```python
from build123d import *

# Parameters (mm, degrees)
SKETCH2_W = 1.05
SKETCH2_H = 10.761
GAP_DEPTH = 3.1


with BuildPart() as part:
    # Sketch1 → Base-Revolve (revolve)
    with BuildSketch(Plane.XY):
        with BuildLine():
            Line((0, 7.1), (0, 10.55))
            Line((0, 10.55), (-2.1, 10.55))
            Line((-2.1, 10.55), (-2.1, 7.1))
            ThreePointArc((-2.1, 7.1), (-1.807106781, 6.392893219), (-1.1, 6.1))
            Line((-1.1, 6.1), (-1, 6.1))
            ThreePointArc((-1, 6.1), (-0.292893219, 6.392893219), (0, 7.1))
        make_face()
    revolve(axis=Axis((-34.925, 0, 0), (1, 0, 0)))

    # Sketch2 → Gap (cut, through all)
    with BuildSketch(Plane(origin=(0, 0, 0), x_dir=(0, -1, 0), z_dir=(-1, 0, 0))):
        with Locations((0, 5.3805)):
            Rectangle(SKETCH2_W, SKETCH2_H)
    extrude(amount=GAP_DEPTH, mode=Mode.SUBTRACT)


solid = part.part
```
Source: CAD feature listing. Evaluate the final solid. Frame: model axes, mm. Coordinates: 2 decimals unless noted, no trailing zeros. Order: outer loops, then holes, each group sorted by start corner. A loop starts at its lowest first (then second) coordinate and runs counter-clockwise, first axis right, second up. Notation, with made-up numbers: M 18.5,36 L 77.5,36 A29 cw 77.5,62 Z; hole C 84.5,53.25 d3. An arc over 180 degrees is marked long. Write each question's results on one line, items separated by ' | '. Start each with the question number.
1) Section query D-D (z = -8). Return the cut outline in (x, y).
2) Draft query along Y for faces 1 (the face through (-1, 0.525, 8)), 2 (the face through (-1, -0.525, 8)), 3 (the face through (0, -2, -7)). Return one class per face: released by +Y, released by -Y, zero draft, split by the parting line, or undercut.
3) Section query B-B (y = 0). Return the cut outline in (x, z).
4) Section query A-A (z = 9). Return the cut outline in (x, y) (3 decimals).
5) Contact query for flat-ended pins moving along their axis: pin 1 Ø2 at (y, z) = (-3.5, 2.5) entering from +X; pin 2 Ø1 at (x, y) = (-0.5, 6.5) entering from +Z; pin 3 Ø1.1 at (x, z) = (-1, 8.5) entering from -Y; pin 4 Ø1.5 at (y, z) = (-1, -7.5) entering from +X. Output: stop coordinate, or through.
6) Line query: line 1 (Y direction, x = -1, z = 0); line 2 (Z direction, x = -1, y = 0); line 3 (Z direction, x = -1.1, y = 2.25). Output: solid intervals per line, ascending. Write a range as from..to.
7) Section query C-C (x = -0.3). Return the cut outline in (y, z) (3 decimals), plus the area to 3 significant figures.
Answers:
1) outline: M -2.1,-6.88 L 0,-6.88 L 0,6.88 L -2.1,6.88 Z
2) face 1: undercut | face 2: undercut | face 3: zero draft
3) outline: M -2.1,-10.55 L 0,-10.55 L 0,-7.1 A1 ccw -1,-6.1 L -1.1,-6.1 A1 ccw -2.1,-7.1 Z
4) outline: M -2.1,-5.505 L 0,-5.505 L 0,-0.525 L -2.1,-0.525 Z; M -2.1,0.525 L 0,0.525 L 0,5.505 L -2.1,5.505 Z
5) pin 1: passes through | pin 2: stops at z = 8.68 | pin 3: stops at y = -6.94 | pin 4: stops at x = 0
6) line 1: y = -10.55..-6.1, 6.1..10.55 | line 2: z = -10.55..-6.1 | line 3: z = -10.31..-5.67, 5.67..10.31
7) outline: M -0.525,6.364 L -0.525,10.537 A10.55 ccw long 0.525,10.537 L 0.525,6.364 A6.386 cw long Z | area: 217 mm^2
